```python
from build123d import *

# Parameters (mm, degrees)
BOSS_EXTRUDE1_DEPTH = 12
SKETCH2_R           = 7.5
CUT_EXTRUDE1_DEPTH  = 50.155365933
SKETCH3_W           = 65
SKETCH3_H           = 3
BOSS_EXTRUDE2_DEPTH = 25
SKETCH4_R           = 1.5
CUT_EXTRUDE2_DEPTH  = 56.229068433


with BuildPart() as part:
    # Sketch1 → Boss-Extrude1 (new, symmetric)
    with BuildSketch(Plane.XY):
        Polygon((32.5, 0), (-32.5, 0), (-32.5, 28), (-12.5, 28), (-12.5, 3), (12.5, 3), (12.5, 28), (32.5, 28), align=None)
    extrude(amount=BOSS_EXTRUDE1_DEPTH, both=True)

    # Sketch2 → Cut-Extrude1 (cut, through all)
    with BuildSketch(Plane.XY.offset(12)):
        with Locations((-22.5, 18)):
            Circle(SKETCH2_R)
    cut_extrude1 = extrude(amount=-CUT_EXTRUDE1_DEPTH, mode=Mode.SUBTRACT)

    # Mirror1: Cut-Extrude1 across plane
    add(cut_extrude1.mirror(Plane(origin=(0, 0, 0), x_dir=(0, 0, 1), z_dir=(1, 0, 0))), mode=Mode.SUBTRACT)

    # Sketch3 → Boss-Extrude2 (add)
    with BuildSketch(Plane.XY.offset(12)):
        with Locations((0, 1.5)):
            Rectangle(SKETCH3_W, SKETCH3_H)
    boss_extrude2 = extrude(amount=BOSS_EXTRUDE2_DEPTH)

    # Sketch4 → Cut-Extrude2 (cut, symmetric)
    with BuildSketch(Plane(origin=(0, 3, 0), x_dir=(1, 0, 0), z_dir=(0, 1, 0))):
        with Locations(Location((-21.25, -24.5, 0), (0, 0, 270))):
            Circle(SKETCH4_R)
        with Locations(Location((21.25, -24.5, 0), (0, 0, 270))):
            Circle(SKETCH4_R)
    cut_extrude2 = extrude(amount=CUT_EXTRUDE2_DEPTH, both=True, mode=Mode.SUBTRACT)

    # Mirror2: Boss-Extrude2, Cut-Extrude2 across plane
    add(boss_extrude2.mirror(Plane.XY))
    add(cut_extrude2.mirror(Plane.XY), mode=Mode.SUBTRACT)


solid = part.part
```
Check sheet for the modelled part. Datum: model origin and axes. Units: mm. A direction names the side the tool comes from. Round coordinates to 2 decimals unless told otherwise and drop trailing zeros. Order: outer loops, then holes, each group sorted by start corner. A loop starts at its lowest first (then second) coordinate and runs counter-clockwise, first axis right, second up. Notation, with made-up numbers: (-39, 12.5) - (13, 12.5) arc R36 cw to (13, 50.5) - close; hole circle Ø10 at (20, 52). An arc over 180 degrees is marked (long way). Answer as CSV lines item,"result". Start each with the question number.
1) Tool access check on faces 1 (the face through (23, 10, 12)), 2 (the face through (28, 23.1, 0.2)), 3 (the face through (12.5, 15, 0)), 4 (the face through (23, 10, -12)). Record the directions out of +Z, -Z, +X, -X, +Y, -Y that give a thin tool (end or side, any length) a straight path to the whole face; none if there is none.
2) Section check C-C (y = 22.5). Record the cut outline in (x, z), then the cut area to 3 significant figures.
3) Scan lines: probe 1 along X at (y, z) = (0.95, -24.5); probe 2 along X at (y, z) = (18.5, 0.5); probe 3 along X at (y, z) = (13, -2.5). Record each from-to range of solid material in increasing order.
4) Draft check along Z on faces 5 (the face through (-20.24, 1.52, -23.39)), 6 (the face through (-22, 10, 12)), 7 (the face through (22.26, 1.52, -23.39)), 8 (the face through (-12.5, 16, 0)). Enter one of: +Z half, -Z half, draft (parallel to the pull), parting line (faces both ways), or undercut.
5) Section check B-B (x = 16.5). Record the cut outline in (y, z), then the cut area to 3 significant figures.
6) Depth check by flat-ended pin: pin 1 (16 mm diameter, centred on x = -17.5, y = 19.5, fed in from -Z); pin 2 (16 mm diameter, centred on x = 19.5, y = 18.5, fed in from +Z). Enter the tip coordinate at first touch or a pass-through.
7) Section check D-D (z = 25). Record the cut outline in (x, y), then the cut area to 3 significant figures.
8) Section check A-A (y = 5). Record the cut outline in (x, z).
Determined:
1,face 1,"+Z, +X, -X, +Y"
1,face 2,"+Z, -Z"
1,face 3,"+Z, -Z, +Y"
1,face 4,"-Z, +X, -X, +Y"
2,outline,"(-32.5, -12) - (-28.5, -12) - (-28.5, 12) - (-32.5, 12) - close; (-16.5, -12) - (-12.5, -12) - (-12.5, 12) - (-16.5, 12) - close; (12.5, -12) - (16.5, -12) - (16.5, 12) - (12.5, 12) - close; (28.5, -12) - (32.5, -12) - (32.5, 12) - (28.5, 12) - close"
2,area,"384 mm^2"
3,probe 1,"-32.5 to -22.75, -19.75 to 19.75, 22.75 to 32.5"
3,probe 2,"-32.5 to -29.98, -15.02 to -12.5, 12.5 to 15.02, 29.98 to 32.5"
3,probe 3,"-32.5 to -28.09, -16.91 to -12.5, 12.5 to 16.91, 28.09 to 32.5"
4,face 5,"undercut"
4,face 6,"+Z half"
4,face 7,"undercut"
4,face 8,"draft"
5,outline,"(0, -37) - (3, -37) - (3, -12) - (13.5, -12) - (13.5, 12) - (3, 12) - (3, 37) - (0, 37) - close; (22.5, -12) - (28, -12) - (28, 12) - (22.5, 12) - close"
5,area,"606 mm^2"
6,pin 1,"z = -12"
6,pin 2,"z = 12"
7,outline,"(-32.5, 0) - (-22.66, 0) - (-22.66, 3) - (-32.5, 3) - close; (-19.84, 0) - (19.84, 0) - (19.84, 3) - (-19.84, 3) - close; (22.66, 0) - (32.5, 0) - (32.5, 3) - (22.66, 3) - close"
7,area,"178 mm^2"
8,outline,"(-32.5, -12) - (-12.5, -12) - (-12.5, 12) - (-32.5, 12) - close; (12.5, -12) - (32.5, -12) - (32.5, 12) - (12.5, 12) - close"
